Design review of the part built by this model. Coordinates are the model's own, in mm. Give positions to 0.01 mm unless a question says otherwise; leave off trailing zeros. Order: outer loops, then holes, each group sorted by start corner. A loop starts at its lowest first (then second) coordinate and runs counter-clockwise, first axis right, second up. Notation, with made-up numbers: (12.25, 28) -> (68.25, 28) arc R24 cw to (68.25, 42) -> close; hole circle Ø6 at (34.5, 49.5). An arc over 180 degrees is marked (long way). One line per item, written item: value.
from build123d import *

# Parameters (mm, degrees)
F0_R     = 250
F1_DEPTH = 2000
F3_R     = 250
F3_R_2   = 50
F4_DEPTH = 25
F6_DEPTH = 2000


with BuildPart() as f1:
    # F0 (on Front) → F1 (new body)
    with BuildSketch(Plane.XZ):
        Circle(F0_R)
    extrude(amount=F1_DEPTH)

    # F3 (on offset) → F4 (cut)
    with BuildSketch(Plane.XZ.offset(1475)):
        Circle(F3_R)
        Circle(F3_R_2, mode=Mode.SUBTRACT)
    extrude(amount=F4_DEPTH, mode=Mode.SUBTRACT)

    # F5 (on face) → F6 (intersect)
    with BuildSketch(Plane.XZ.offset(2000)):
        with BuildLine():
            ThreePointArc((21.7889356869, 249.0486745229), (10.9048468413, 249.7620553955), (0, 250))
            Line((0, 250), (0, 25))
            ThreePointArc((0, 25), (1.0904846841, 24.9762055395), (2.1788935687, 24.9048674523))
            Line((2.1788935687, 24.9048674523), (21.7889356869, 249.0486745229))
        make_face()
    extrude(amount=-F6_DEPTH, mode=Mode.INTERSECT)


solid = f1.part
Item 1: Add section A-A on x = 15.75. Give the boundary of the cut face in (y, z), plus the area to 3 significant figures.
Returned:
outline: (-2000, 180.02) -> (-1500, 180.02) -> (-1500, 249.5) -> (-2000, 249.5) -> close; (-1475, 180.02) -> (0, 180.02) -> (0, 249.5) -> (-1475, 249.5) -> close
area: 137,000 mm²
Item 2: To check wall thickness, follow line 1 along Y through (x, z) = (2.5, 126); line 2 along X through (y, z) = (-731.5, 49.5); line 3 along Z through (x, y) = (1.75, -1548). State the ranges of each line that lie inside material, in increasing order. Write a range as from..to.
Returned:
line 1: -2000..-1500, -1475..0
line 2: 0..4.33
line 3: 24.94..249.99
Item 3: Add section B-B on z = 150. Give the boundary of the cut face in (x, y).
Returned:
outline: (0, -2000) -> (13.12, -2000) -> (13.12, -1500) -> (0, -1500) -> close; (0, -1475) -> (13.12, -1475) -> (13.12, 0) -> (0, 0) -> close
Item 4: Clearance check with flat-ended pins moving along their axes: P1, Ø6, axis at x = 6, z = 73, coming from the +Y side; P2, Ø6, axis at x = 16.5, y = -1750.5, coming from the +Z side; P3, Ø6, axis at x = 9.5, y = -240.5, coming from the +Z side; P4, Ø2, axis at y = -499, z = 69, coming from the +X side. State where each tip first meets the part, or that it passes through.
Returned:
P1: y = 0
P2: z = 249.64
P3: z = 249.92
P4: x = 6.12
Item 5: Add section C-C on y = -1520. Give the boundary of the cut face in (x, z), plus the area to 3 significant figures.
Returned:
outline: (0, 25) arc R25 cw to (2.18, 24.9) -> (21.79, 249.05) arc R250 ccw to (0, 250) -> close
area: 2,700 mm²
